Can you work these out from the model? Positions are in its coordinate system, mm. Face numbers are marked on the shaded views. A direction names the side the tool comes from. Round coordinates to 2 decimals unless told otherwise and drop trailing zeros. Order: outer loops, then holes, each group sorted by start corner. A loop starts at its lowest first (then second) coordinate and runs counter-clockwise, first axis right, second up.
Q1. If we section it at A-A (y = -17): Please give me the cut outline in (x, z), plus the area to 3 significant figures.
Q2. If we section it at D-D (y = -30.5): Please give me the cut outline in (x, z), plus the area to 3 significant figures.
Q3. For the marked faces 1, 2 and 3, which set-ups out of +Z, -Z, +X, -X, +Y, -Y let a thin tool reach every point of the face, with its end or its side?
Q4. If we section it at C-C (z = 25.5): Please give me the cut outline in (x, y) (3 decimals).
Q5. If we section it at B-B (z = -30.5): Please give me the cut outline in (x, y), plus the area to 3 significant figures.
Q6. If I drill on line 1 (X direction, y = -27, z = -31.5); line 2 (Z direction, x = 18, y = -26); line 3 (Y direction, x = 33, z = 6), over which ranges is the centre line in solid material (lowest first)?
Q7. Will these pins go through, and if not, where does the flat tip stop? P1, Ø10, axis at y = -34, z = -29.5, coming from the -X side; P2, Ø5, axis at x = -16.5, y = -13, coming from the +Z side; P3, Ø14, axis at y = -24.5, z = -28.5, coming from the +X side; P4, Ø6, axis at x = -29.5, y = -17, coming from the +Z side.
Q8. We'd pull the mould along Z, two halves only. Please class the marked faces 4, 5 and 6: pulls with the +Z half, pulls with the -Z half, needs draft (parallel to the pull), parting line crosses it, or undercut.
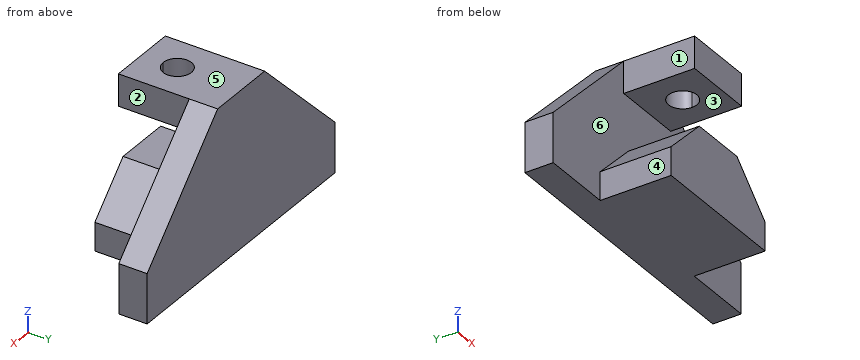
from build123d import *

# Parameters (mm, degrees)
F1_DEPTH = 12.7
F3_DEPTH = 31.75
F4_W     = 31.75
F4_H     = 14.2875
F5_DEPTH = 31.75
F7_DEPTH = 25.4


with BuildPart() as f1:
    # F0 (on Front) → F1 (new body)
    with BuildSketch(Plane.XZ):
        Polygon((-57.3339015245, -14.512266928), (-57.3339015245, -36.737266928), (69.6660984755, -36.737266928), (69.6660984755, -14.512266928), (22.0410984755, 33.112733072), (-9.7089015245, 33.112733072), align=None)
    extrude(amount=F1_DEPTH)

    # F2 (on face) → F3 (join)
    with BuildSketch(Plane.XZ.offset(12.7)):
        Polygon((-25.5839015245, -36.737266928), (37.9160984755, -36.737266928), (37.9160984755, -24.037266928), (18.8660984755, -24.037266928), (18.8660984755, -4.987266928), (-6.5339015245, -4.987266928), (-6.5339015245, -24.037266928), (-25.5839015245, -24.037266928), align=None)
        Polygon((18.8660984755, -24.037266928), (37.9160984755, -24.037266928), (18.8660984755, -4.987266928), align=None)
        Polygon((-6.5339015245, -4.987266928), (-25.5839015245, -24.037266928), (-6.5339015245, -24.037266928), align=None)
    extrude(amount=F3_DEPTH)

    # F4 (on face) → F5 (join)
    with BuildSketch(Plane.XZ.offset(12.7)):
        with Locations((6.1660984755, 25.968983072)):
            Rectangle(F4_W, F4_H)
    extrude(amount=F5_DEPTH)

    # F6 (on face) → F7 (cut)
    with BuildSketch(Plane.XY.offset(33.112733072)):
        with BuildLine():
            ThreePointArc((6.1660984755, -34.925), (10.656226536, -33.0651280605), (12.5160984755, -28.575))
            ThreePointArc((12.5160984755, -28.575), (1.6759704149, -24.0848719395), (6.1660984755, -34.925))
        make_face()
    extrude(amount=-F7_DEPTH, mode=Mode.SUBTRACT)


solid = f1.part
Solution:
1. outline: (-25.58, -36.74) - (37.92, -36.74) - (37.92, -24.04) - (18.87, -4.99) - (-6.53, -4.99) - (-25.58, -24.04) - close; (-9.71, 18.83) - (22.04, 18.83) - (22.04, 33.11) - (-9.71, 33.11) - close
1. area: 2,110 mm2
2. outline: (-25.58, -36.74) - (37.92, -36.74) - (37.92, -24.04) - (18.87, -4.99) - (-6.53, -4.99) - (-25.58, -24.04) - close; (-9.71, 18.83) - (0.11, 18.83) - (0.11, 33.11) - (-9.71, 33.11) - close; (12.22, 18.83) - (22.04, 18.83) - (22.04, 33.11) - (12.22, 33.11) - close
2. area: 1,930 mm2
3. face 1: +Z, -X, -Y
3. face 2: +Z, +X, -Y
3. face 3: +X, -X, -Y
4. outline: (-17.322, -12.7) - (-9.709, -12.7) - (-9.709, -44.45) - (22.041, -44.45) - (22.041, -12.7) - (29.654, -12.7) - (29.654, 0) - (-17.322, 0) - close; hole circle Ø12.7 at (6.166, -28.575)
5. outline: (-57.33, -12.7) - (-25.58, -12.7) - (-25.58, -44.45) - (37.92, -44.45) - (37.92, -12.7) - (69.67, -12.7) - (69.67, 0) - (-57.33, 0) - close
5. area: 3,630 mm2
6. line 1: x = -25.58 to 37.92
6. line 2: z = -36.74 to -4.99, 18.83 to 33.11
6. line 3: y = -12.7 to 0
7. P1: stops at x = -25.58
7. P2: stops at z = 28.8
7. P3: stops at x = 37.92
7. P4: passes through
8. face 4: needs draft
8. face 5: pulls with the +Z half
8. face 6: undercut
